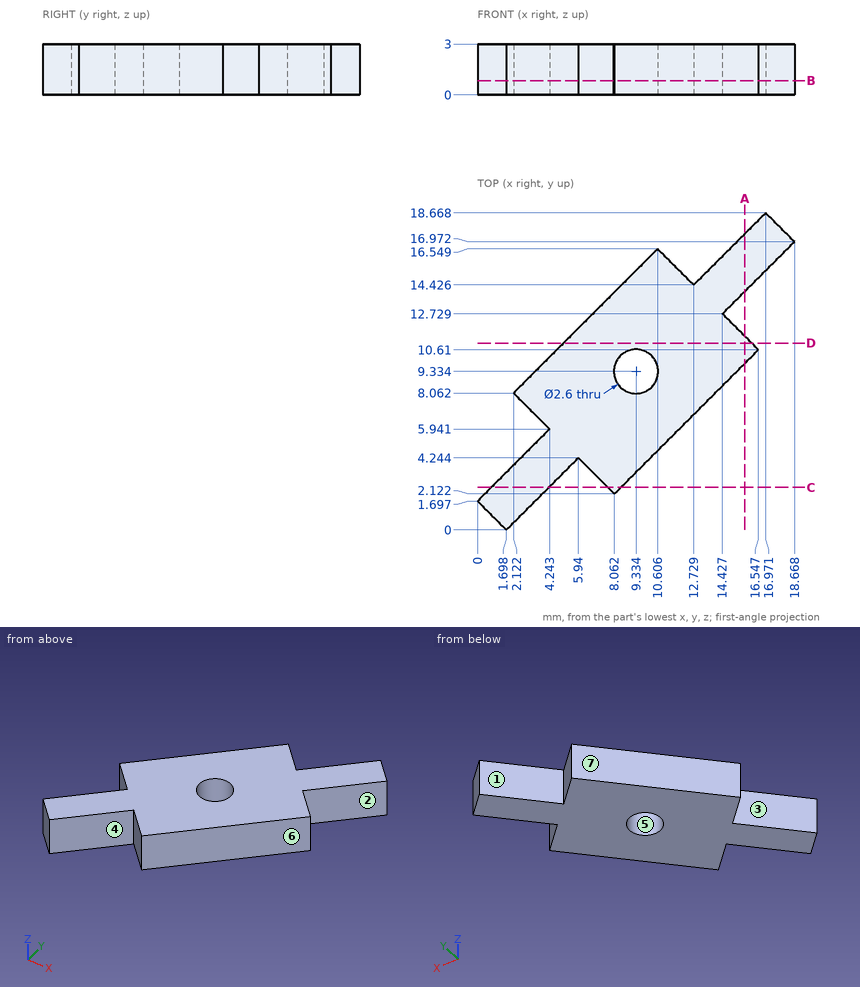
Part print with two shaded views. Sizes in mm from the minimum x, y, z corner. A direction names the side the tool comes from. Give positions to 0.01 mm unless a question says otherwise; leave off trailing zeros. Order: outer loops, then holes, each group sorted by start corner. A loop starts at its lowest first (then second) coordinate and runs counter-clockwise, first axis right, second up. Notation, with made-up numbers: (14, 26) - (22, 26) arc R24 ccw to (22, 43) - close; hole circle Ø8 at (39.5, 49). An arc over 180 degrees is marked (long way). Write each question's results on one line, items separated by ' | '.
1. Saw through at B-B on z = 0.85. List the corners of the cut face in (x, y) (1 decimal).
Calculated:
outline: (0, 1.7) - (1.7, 0) - (5.9, 4.2) - (8.1, 2.1) - (16.5, 10.6) - (14.4, 12.7) - (18.7, 17) - (17, 18.7) - (12.7, 14.4) - (10.6, 16.5) - (2.1, 8.1) - (4.2, 5.9) - close; hole circle Ø2.6 at (9.3, 9.3)
2. Pull direction X, two halves, no side cores. Call the marked faces 5, 6 and 7: released by +X, released by -X, zero draft, split by the parting line, or undercut.
Calculated:
face 5: undercut | face 6: released by +X | face 7: released by -X
3. Saw through at A-A on x = 15.75. List the corners of the cut face in (y, z).
Calculated:
outline: (9.81, 0) - (11.41, 0) - (11.41, 3) - (9.81, 3) - close; (14.05, 0) - (17.45, 0) - (17.45, 3) - (14.05, 3) - close
4. Saw through at C-C on y = 2.5. List the corners of the cut face in (x, z) (1 decimal).
Calculated:
outline: (0.8, 0) - (4.2, 0) - (4.2, 3) - (0.8, 3) - close; (7.7, 0) - (8.4, 0) - (8.4, 3) - (7.7, 3) - close
5. 3-axis set-ups, long thin cutter, end or side, ignore diameter. For the marked faces 1, 2, 3 and 4: which of +Z, -Z, +X, -X, +Y, -Y reach the whole face in a straight line?
Calculated:
face 1: +Z, -Z, +Y | face 2: +Z, -Z, +X | face 3: +Z, -Z, -X | face 4: +Z, -Z, -Y
6. Probe L1, parallel to X at y = 9, z = 0.3 (1 decimal); L2, parallel to Y at x = 3.5, z = 2 (1 decimal); L3, parallel to Y at x = 6, z = 0.25 (1 decimal). List the from-to ranges inside material, lowest first. Write a range as from..to.
Calculated:
L1: x = 3.1..8.1, 10.6..14.9 | L2: y = 1.8..5.2, 6.7..9.4 | L3: y = 4.2..11.9
7. Saw through at D-D on y = 11. List the corners of the cut face in (x, z), and give its area (3 significant figures).
Calculated:
outline: (5.06, 0) - (16.16, 0) - (16.16, 3) - (5.06, 3) - close | area: 33.3 mm2
8. Pin check, flat tip, straight feed: pin 1 (1.6 mm diameter, centred on x = 9.33, y = 9.33, fed in from +Z). Stop position of the tip, or through.
Calculated:
pin 1: passes through
